```python
from build123d import *

# Parameters (mm, degrees)
F0_W         = 20
F0_H         = 50
F0_R         = 2.5
F1_DEPTH     = 1
F2_T         = -1.5
F3_T         = 1
F3_T3_DEPTH  = 23.5635083269
F3_T5_DEPTH  = 2.5
F3_T7_DEPTH  = 23.5635083269
F3_T9_DEPTH  = 19
F3_T11_DEPTH = 49
F3_T14_ANGLE = 302.0899512573


# Not quite as in the source:
# - a shell that OpenCascade refuses in one call is made with other operations: the cavity is built on its own and cut out


with BuildPart() as f1:
    # F0 (on Front) → F1 (new body, symmetric)
    with BuildSketch(Plane.XZ):
        Rectangle(F0_W, F0_H)
        with Locations((5, 0)):
            Circle(F0_R, mode=Mode.SUBTRACT)
    extrude(amount=F1_DEPTH, both=True)

    # F2
    f2_openings = [f1.faces().sort_by_distance(p)[0] for p in [
        (-0.100141, -1, 0),
    ]]
    offset(amount=F2_T, openings=f2_openings, kind=Kind.INTERSECTION)

    # F3: shell of thickness 1, made by hand


with BuildPart() as f3_core1:
    # F3_t2: copy of F1
    add(f1.part)

    # the walls: a layer under each face that stays
    f3_faces = [f3_core1.faces().sort_by_distance(p)[0] for p in [
        (10, 0, 0),
        (0, 0, -25),
        (-10, 0, 0),
        (0, 0, 25),
        (2.5, 0, 0),
        (-8.5714285714, -1, -21.4285714286),
        (8.5, -0.75, 12.7182458366),
        (8.5, -0.75, -12.7182458366),
        (0, -0.75, -23.5),
        (-8.5, -0.75, 0),
        (1, -0.75, 0),
        (0, -0.75, 23.5),
        (0, -0.5, 0),
    ]]
    thicken(f3_faces, amount=-F3_T, mode=Mode.SUBTRACT)

    # F3_s4 → F3_t3 (cut)
    with BuildSketch(Plane.XY.offset(0.9364916731)):
        Polygon((8.49, -0.51), (9.5, -0.5), (9.5, 0.5), (8.5, 0.5), align=None)
    extrude(amount=F3_T3_DEPTH, mode=Mode.SUBTRACT)

    # F3_s6 → F3_t5 (cut)
    with BuildSketch(Plane.XZ.offset(-0.5)):
        Polygon((8.49, 23.49), (9.5, 23.5), (9.5, 24.5), (8.5, 24.5), align=None)
        Polygon((8.49875, 1.9413329023), (9.5, 1.9364916731), (9.5, -1.9364916731), (7.625, 1.4523687548), align=None)
        Polygon((8.49, -23.49), (9.5, -23.5), (9.5, -24.5), (8.5, -24.5), align=None)
        Polygon((8.49875, -1.9413329023), (9.5, -1.9364916731), (9.5, 1.9364916731), (7.625, -1.4523687548), align=None)
        Polygon((-8.49, -23.49), (-8.5, -24.5), (-9.5, -24.5), (-9.5, -23.5), align=None)
        Polygon((-8.49, 23.49), (-9.5, 23.5), (-9.5, 24.5), (-8.5, 24.5), align=None)
    extrude(amount=F3_T5_DEPTH, mode=Mode.SUBTRACT)

    # F3_s8 → F3_t7 (cut)
    with BuildSketch(Plane.XY.offset(-24.5)):
        Polygon((8.49, -0.51), (9.5, -0.5), (9.5, 0.5), (8.5, 0.5), align=None)
    extrude(amount=F3_T7_DEPTH, mode=Mode.SUBTRACT)

    # F3_s10 → F3_t9 (cut)
    with BuildSketch(Plane.YZ.offset(-9.5)):
        Polygon((-0.51, -23.49), (-0.5, -24.5), (0.5, -24.5), (0.5, -23.5), align=None)
        Polygon((-0.51, 23.49), (-0.5, 24.5), (0.5, 24.5), (0.5, 23.5), align=None)
    extrude(amount=F3_T9_DEPTH, mode=Mode.SUBTRACT)

    # F3_s12 → F3_t11 (cut)
    with BuildSketch(Plane.XY.offset(-24.5)):
        Polygon((-8.49, -0.51), (-9.5, -0.5), (-9.5, 0.5), (-8.5, 0.5), align=None)
    extrude(amount=F3_T11_DEPTH, mode=Mode.SUBTRACT)

    # F3_s13 → F3_t14 (revolve, cut)
    with BuildSketch(Plane(origin=(1.171875, 0, 2.1180377675), x_dir=(0, 1, 0), z_dir=(0.4841229183, 0, 0.875))):
        Polygon((-0.51, -8.385), (-0.5, -7.375), (0.5, -7.375), (0.5, -8.375), align=None)
    revolve(axis=Axis((5, -0.5, 0), (0, 1, 0)), revolution_arc=F3_T14_ANGLE, mode=Mode.SUBTRACT)


with BuildPart() as f1_1:
    add(f1.part)

    # what is left inside the walls is the cavity
    f3_cavity = [f3_core1.part.solids().sort_by_distance(p)[0] for p in [
        (0, 0.99, -8),
    ]]
    add(f3_cavity, mode=Mode.SUBTRACT)


solid = f1_1.part
```
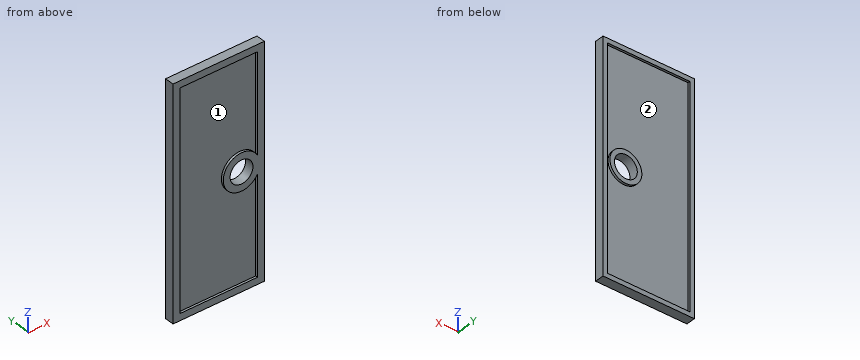
For this review, take the finished solid that the model builds, in its own axes (mm). Face numbers are marked on the shaded views. A direction names the side the tool comes from. Coordinates: 2 decimals unless noted, no trailing zeros. Write each loop counter-clockwise with the first axis right and the second up, starting at its lowest first coordinate (ties: lowest second). Pieces come first, ordered by that corner, then holes. Notation, with made-up numbers: (56.5, 83.5) -> (113.5, 83.5) arc R24 cw to (113.5, 110.5) -> close; hole circle Ø5 at (65.25, 5.5). An arc over 180 degrees is marked (long way). Put each result on its own line as item: value.
Q1. Take a section at A-A, the plane z = 0. State the section outline as (x, y) points, then the cut area to 4 significant figures.
From the geometry:
outline: (-10, -1) -> (-8.5, -1) -> (-8.5, -0.5) -> (1, -0.5) -> (1, -1) -> (2.5, -1) -> (2.5, 1) -> (1.5, 1) -> (1.5, 0.5) -> (-9, 0.5) -> (-9, 1) -> (-10, 1) -> close; (7.5, -1) -> (10, -1) -> (10, 1) -> (9, 1) -> (9, 0.5) -> (8.5, 0.5) -> (8.5, 1) -> (7.5, 1) -> close
area: 19.75 mm2
Q2. Wall thickness on L1, parallel to Z at x = 5, y = 0.65; L2, parallel to Z at x = 5, y = -0.25; L3, parallel to X at y = 0.95, z = -11: over which ranges is each line inside the solid? List them lowest first.
From the geometry:
L1: z = -25 to -24, -3.5 to -2.5, 2.5 to 3.5, 24 to 25
L2: z = -25 to -2.5, 2.5 to 25
L3: x = -10 to -9, 9 to 10
Q3. Take a section at C-C, the plane y = -0.15. State the section outline as (x, z) points.
From the geometry:
outline: (-10, -25) -> (10, -25) -> (10, 25) -> (-10, 25) -> close; hole circle Ø5 at (5, 0)
Q4. Clearance check with flat-ended pins moving along their axes: pin 1 Ø1.5 at (x, z) = (6.5, 16.5) entering from +Y; pin 2 Ø1.5 at (x, z) = (-1, -11) entering from -Y. State where each tip first meets the part, or that it passes through.
From the geometry:
pin 1: stops at y = 0.5
pin 2: stops at y = -0.5
Q5. Tool access review of the marked faces 1 and 2: name each direction out of +Z, -Z, +X, -X, +Y, -Y from which nothing blocks a thin tool from reaching the whole face with its end or side.
From the geometry:
face 1: -Y
face 2: +Y
Q6. Take a section at B-B, the plane x = 5. State the section outline as (y, z) points, then the cut area to 3 significant figures.
From the geometry:
outline: (-1, -25) -> (1, -25) -> (1, -24) -> (0.5, -24) -> (0.5, -3.5) -> (1, -3.5) -> (1, -2.5) -> (-1, -2.5) -> (-1, -4) -> (-0.5, -4) -> (-0.5, -23.5) -> (-1, -23.5) -> close; (-1, 2.5) -> (1, 2.5) -> (1, 3.5) -> (0.5, 3.5) -> (0.5, 24) -> (1, 24) -> (1, 25) -> (-1, 25) -> (-1, 23.5) -> (-0.5, 23.5) -> (-0.5, 4) -> (-1, 4) -> close
area: 50.0 mm2
Q7. Take a section at D-D, the plane x = -1.75. State the section outline as (y, z) points, then the cut area to 3 significant figures.
From the geometry:
outline: (-1, -25) -> (1, -25) -> (1, -24) -> (0.5, -24) -> (0.5, 24) -> (1, 24) -> (1, 25) -> (-1, 25) -> (-1, 23.5) -> (-0.5, 23.5) -> (-0.5, -23.5) -> (-1, -23.5) -> close
area: 52.5 mm2
